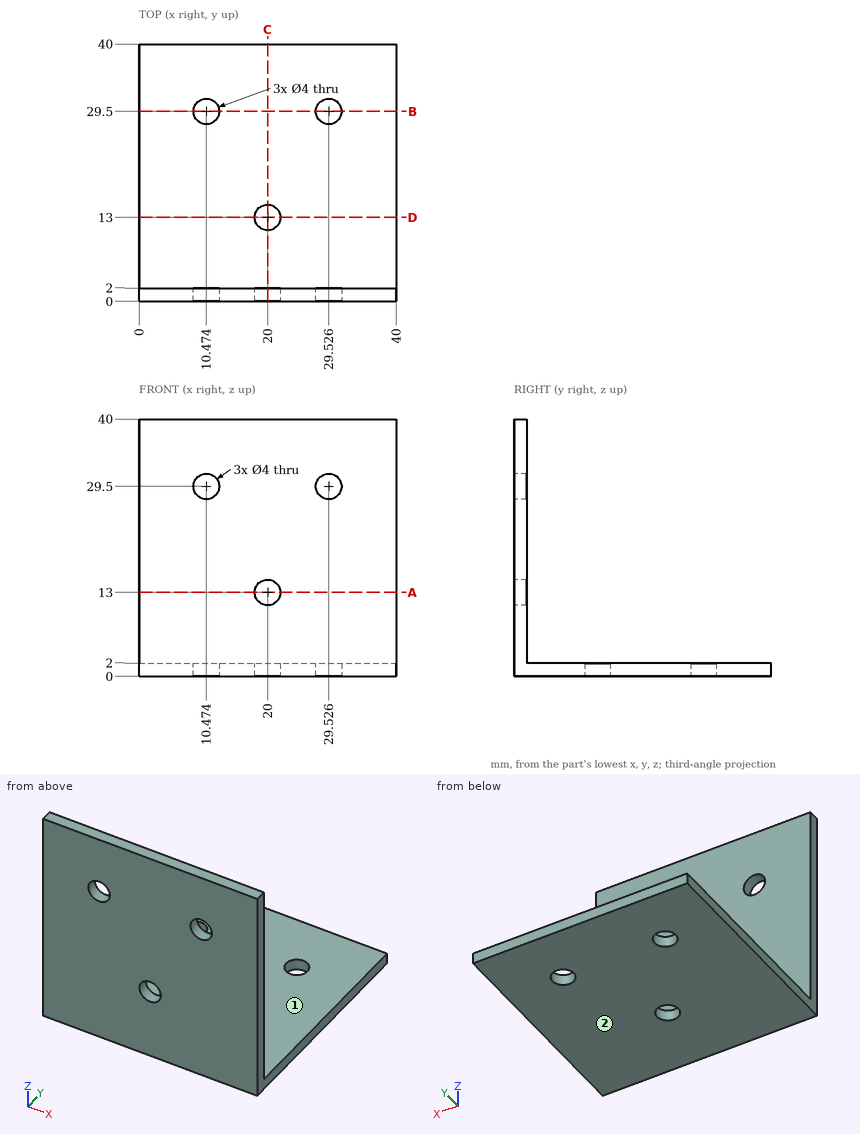
Study the drawing (mm; zero at the part's minimum x, y, z) and answer. A direction names the side the tool comes from. Round coordinates to 2 decimals unless told otherwise and drop trailing zeros. Write each loop counter-clockwise with the first axis right and the second up, starting at its lowest first coordinate (ties: lowest second). Pieces come first, ordered by that corner, then holes. Notation, with made-up numbers: (22.5, 20.5) - (77.5, 20.5) arc R23 ccw to (77.5, 44.5) - close; hole circle Ø2 at (9, -7). An arc over 180 degrees is marked (long way). Use a Markdown table: item, result. Add a question column.
1. A tool of negligible diameter and unlimited length cuts with its end or side. For the marked faces 1 and 2, from which of +Z, -Z, +X, -X, +Y, -Y can it reach the whole face along a straight path? Write none if from no direction.
2. Flat-ended cylindrical pins translate along their axes: P1, Ø3, axis at x = 10.47, y = 29.5, coming from the -Z side (3 decimals); P2, Ø6.5, axis at x = 29.53, y = 29.5, coming from the +Z side; P3, Ø8, axis at x = 20.5, z = 6.5, coming from the -Y side; P4, Ø5, axis at x = 29.53, z = 29.5, coming from the +Y side. Find the tip coordinate at first contact, or state that the pin passes through.
3. The part is cut by section C-C (x = 20). Write down the section's boundary in (y, z), and give its area (3 significant figures).
4. The part is cut by section A-A (z = 13). Write down the section's boundary in (x, y), and give its area (3 significant figures).
5. Consider line 1 (Z direction, x = 20, y = 1.3); line 2 (Y direction, x = 33, z = 9.5). Determine where each line is inside the solid, lowest interval first.
6. The part is cut by section B-B (y = 29.5). Write down the section's boundary in (x, z), and give its area (3 significant figures).
Reported:
| question | item | result |
|---|---|---|
| 1 | face 1 | +Z, +X, -X, +Y |
| 1 | face 2 | -Z, +X, -X, +Y, -Y |
| 2 | P1 | through |
| 2 | P2 | z = 2 |
| 2 | P3 | y = 0 |
| 2 | P4 | y = 2 |
| 3 | outline | (0, 0) - (11, 0) - (11, 2) - (2, 2) - (2, 11) - (0, 11) - close; (0, 15) - (2, 15) - (2, 40) - (0, 40) - close; (15, 0) - (40, 0) - (40, 2) - (15, 2) - close |
| 3 | area | 140 mm^2 |
| 4 | outline | (0, 0) - (18, 0) - (18, 2) - (0, 2) - close; (22, 0) - (40, 0) - (40, 2) - (22, 2) - close |
| 4 | area | 72.0 mm^2 |
| 5 | line 1 | 0 to 11, 15 to 40 |
| 5 | line 2 | 0 to 2 |
| 6 | outline | (0, 0) - (8.47, 0) - (8.47, 2) - (0, 2) - close; (12.47, 0) - (27.53, 0) - (27.53, 2) - (12.47, 2) - close; (31.53, 0) - (40, 0) - (40, 2) - (31.53, 2) - close |
| 6 | area | 64.0 mm^2 |
